Check sheet for the modelled part. Datum: model origin and axes. Units: mm. Face numbers are marked on the shaded views. A direction names the side the tool comes from. Give positions to 0.01 mm unless a question says otherwise; leave off trailing zeros. Loops run counter-clockwise (first coordinate to the right, second up) from the corner with the lowest first, then second, coordinate; pieces in that order, holes last. Notation, with made-up numbers: M -33.75,13 L -1.75,13 A14 cw -1.75,37 Z; hole C 76.25,-27.75 d11. An arc over 180 degrees is marked long. Write each question's results on one line, items separated by ' | '. Start each with the question number.
1. Draft check along Y on the marked faces 4, 5 and 6. Enter one of: pulls with the +Y half, pulls with the -Y half, needs draft (parallel to the pull), parting line crosses it, or undercut.
2. Sectioned sample at C-C on z = 119.5. Record the cut outline in (x, y), and give its area (3 significant figures).
3. Material ranges on line 1 along Z through (x, y) = (-6, 0); line 2 along Y through (x, z) = (-67, 17); line 3 along Z through (x, y) = (-38, 40), recorded low to high.
4. Go/stop test with a flat-tipped pin: pin 1 (1.5 mm diameter, centred on y = -11, z = 38, fed in from +X). Record where the tip stops, or that it passes through.
5. Sectioned sample at B-B on x = -68.5. Record the cut outline in (y, z), and give its area (3 significant figures).
6. Tool access check on the marked faces 1, 2 and 3. Record the directions out of +Z, -Z, +X, -X, +Y, -Y that give a thin tool (end or side, any length) a straight path to the whole face; none if there is none.
7. Sectioned sample at A-A on y = 0. Record the cut outline in (x, z), and give its area (3 significant figures).
8. Sectioned sample at D-D on y = 65. Record the cut outline in (x, z), and give its area (3 significant figures).
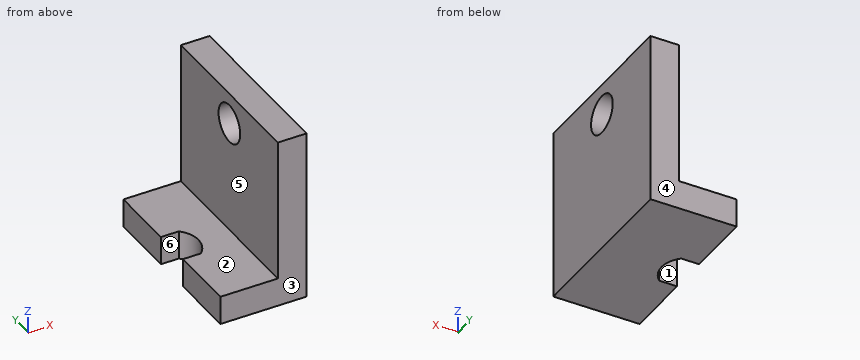
```python
from build123d import *

# Parameters (mm, degrees)
F1_DEPTH = 76.2
F2_R     = 17.019042
F3_DEPTH = 38.1
F5_DEPTH = 25.4


with BuildPart() as f1:
    # F0 (on Front) → F1 (new body, symmetric)
    with BuildSketch(Plane.XZ):
        Polygon((0, 0), (0, 152.4), (-25.4, 152.4), (-25.4, 25.4), (-76.2, 25.4), (-76.2, 0), align=None)
    extrude(amount=F1_DEPTH, both=True)

    # F2 (on face) → F3 (cut)
    with BuildSketch(Plane.YZ):
        with Locations((0, 124.789342)):
            Circle(F2_R)
    extrude(amount=-F3_DEPTH, mode=Mode.SUBTRACT)

    # F4 (on face) → F5 (cut, symmetric)
    with BuildSketch(Plane.XY.offset(25.4)):
        with BuildLine():
            Line((-76.2, -17.294263), (-60.396418, -17.294263))
            ThreePointArc((-60.396418, -17.294263), (-52.772565, 0), (-60.396418, 17.294263))
            Line((-60.396418, 17.294263), (-76.2, 17.294263))
            Line((-76.2, 17.294263), (-76.2, -17.294263))
        make_face()
    extrude(amount=F5_DEPTH, both=True, mode=Mode.SUBTRACT)


solid = f1.part
```
Output values:
1) face 4: pulls with the +Y half | face 5: needs draft | face 6: undercut
2) outline: M -25.4,-76.2 L 0,-76.2 L 0,-16.18 L -25.4,-16.18 Z; M -25.4,16.18 L 0,16.18 L 0,76.2 L -25.4,76.2 Z | area: 3,050 mm2
3) line 1: 0 to 107.77, 141.81 to 152.4 | line 2: -76.2 to -17.29, 17.29 to 76.2 | line 3: 0 to 25.4
4) pin 1: x = 0
5) outline: M -76.2,0 L -17.29,0 L -17.29,25.4 L -76.2,25.4 Z; M 17.29,0 L 76.2,0 L 76.2,25.4 L 17.29,25.4 Z | area: 2,990 mm2
6) face 1: +Z, -Z, -X | face 2: +Z, -X, +Y, -Y | face 3: +Z, -Z, +X, -X, -Y
7) outline: M -52.77,0 L 0,0 L 0,107.77 L -25.4,107.77 L -25.4,25.4 L -52.77,25.4 Z; M -25.4,141.81 L 0,141.81 L 0,152.4 L -25.4,152.4 Z | area: 3,700 mm2
8) outline: M -76.2,0 L 0,0 L 0,152.4 L -25.4,152.4 L -25.4,25.4 L -76.2,25.4 Z | area: 5,160 mm2
